Geometry: final body of the model. Coordinates: model frame, mm. A direction names the side the tool comes from. Give positions to 0.01 mm unless a question says otherwise; leave off trailing zeros. Order: outer loops, then holes, each group sorted by start corner. A loop starts at its lowest first (then second) coordinate and runs counter-clockwise, first axis right, second up. Notation, with made-up numbers: (37, -7) -> (46, -7) arc R24 ccw to (46, 18) -> close; hole circle Ø8 at (16, -38). An arc over 180 degrees is marked (long way). Write item = value, one per line.
```python
from build123d import *

# Parameters (mm, degrees)
SKETCH_1_W           = 174.15
SKETCH_1_H           = 108
EXTRUDE_1_DEPTH      = 63
CUT_EXTRUDE_2_DEPTH  = 174.15
CUT_EXTRUDE_3_REACH  = 122.279
SKETCH_6_W           = 2
SKETCH_6_H           = 108
SKETCH_7_W           = 96
SKETCH_7_H           = 50.25
CUT_EXTRUDE_5_DEPTH  = 168.15
SKETCH_8_W           = 87.5
SKETCH_8_H           = 4.75
CUT_EXTRUDE_6_DEPTH  = 168.15
SKETCH_10_W          = 168.15
SKETCH_10_H          = 87.5
CUT_EXTRUDE_8_DEPTH  = 59
SKETCH_12_W          = 168.15
SKETCH_12_H          = 96
EXTRUDE_2_DEPTH      = 2
SKETCH_15_W          = 25
SKETCH_15_H          = 70
SKETCH_15_W_2        = 55
SKETCH_15_H_2        = 20
SKETCH_15_W_3        = 44.398131355
SKETCH_15_H_3        = 87.5
CUT_EXTRUDE_9_DEPTH  = 2
SKETCH_16_W          = 25
SKETCH_16_H          = 96
SKETCH_16_W_2        = 32.283516817
CUT_EXTRUDE_10_DEPTH = 2
SKETCH_17_W          = 2
SKETCH_17_H          = 96
EXTRUDE_3_DEPTH      = 5
SKETCH_18_W          = 2
SKETCH_18_H          = 87.5
EXTRUDE_4_DEPTH      = 5
SKETCH_19_W          = 100
SKETCH_19_H          = 18
CUT_EXTRUDE_11_DEPTH = 6
CUT_EXTRUDE_12_REACH = 154.365
EXTRUDE_5_REACH      = 154.365
SKETCH_23_W          = 65.205598619
SKETCH_23_H          = 48.744694075
CUT_EXTRUDE_13_DEPTH = 2
CUT_EXTRUDE_START    = -63
CUT_EXTRUDE_14_DEPTH = 63
SKETCH_28_W          = 2
SKETCH_28_H          = 4.25
EXTRUDE_6_DEPTH      = 4.75
SKETCH_31_W          = 13
SKETCH_31_H          = 55
CUT_EXTRUDE_15_DEPTH = 10
SKETCH_34_W          = 103.070926165
SKETCH_34_H          = 3
CUT_EXTRUDE_16_DEPTH = 143.15
SKETCH_37_W          = 0.5
SKETCH_37_H          = 0.5
EXTRUDE_7_DEPTH      = 1
EXTRUDE_7_2_DEPTH    = 1
EXTRUDE_7_3_DEPTH    = 1
EXTRUDE_7_4_DEPTH    = 1
EXTRUDE_7_5_DEPTH    = 1
EXTRUDE_7_6_DEPTH    = 1
EXTRUDE_7_7_DEPTH    = 1
SKETCH_40_W          = 0.5
SKETCH_40_H          = 0.5
EXTRUDE_8_DEPTH      = 1
SKETCH_42_W          = 2.002594571
SKETCH_42_H          = 94
EXTRUDE_9_DEPTH      = 63


with BuildPart() as part:
    # Sketch 1 → Extrude 1 (new body)
    with BuildSketch(Plane(origin=(0, 0, 0), x_dir=(1, 0, 0), z_dir=(0, 1, 0))):
        Rectangle(SKETCH_1_W, SKETCH_1_H)
    extrude(amount=EXTRUDE_1_DEPTH)

    # Sketch 5 → Cut-Extrude 2 (cut)
    with BuildSketch(Plane.ZY.offset(87.075)):
        Polygon((-48, 0), (-47.75, 0), (-47.75, 2.75), (-45.75, 2.75), (-45.75, 4.75), (-52.25, 4.75), (-52.25, 2.75), (-50.25, 2.75), (-50.25, 0), (-50, 0), (-50, 3), (-52, 3), (-52, 4.5), (-46, 4.5), (-46, 3), (-48, 3), align=None)
        Polygon((-50, 0), (-48, 0), (-48, 3), (-46, 3), (-46, 4.5), (-52, 4.5), (-52, 3), (-50, 3), align=None)
        Polygon((50, 3), (50, 0), (50.25, 0), (50.25, 2.75), (52.25, 2.75), (52.25, 4.75), (45.75, 4.75), (45.75, 2.75), (47.75, 2.75), (47.75, 0), (48, 0), (48, 3), (46, 3), (46, 4.5), (52, 4.5), (52, 3), align=None)
        Polygon((48, 0), (50, 0), (50, 3), (52, 3), (52, 4.5), (46, 4.5), (46, 3), (48, 3), align=None)
    extrude(amount=-CUT_EXTRUDE_2_DEPTH, mode=Mode.SUBTRACT)

    # Cut-Extrude 3: up to this face of the body (flat: up to its plane)
    cut_extrude_3_end = Plane(part.part.faces().sort_by_distance((0, 4.75, 49))[0])
    # Sketch 6 → Cut-Extrude 3 (cut, up to the picked face)
    with BuildSketch(Plane.XZ, mode=Mode.PRIVATE) as cut_extrude_3_sk1:
        with Locations((-86.075, 0)):
            Rectangle(SKETCH_6_W, SKETCH_6_H)
    cut_extrude_3_tool1 = split(extrude(cut_extrude_3_sk1.sketch, amount=-CUT_EXTRUDE_3_REACH, mode=Mode.PRIVATE), bisect_by=cut_extrude_3_end, keep=Keep.BOTH, mode=Mode.PRIVATE)
    add(cut_extrude_3_tool1.solids().sort_by(Axis((-86.075, 0, 0), (0, 1, 0)))[0], mode=Mode.SUBTRACT)

    # Sketch 7 → Cut-Extrude 5 (cut)
    with BuildSketch(Plane(origin=(87.075, 0, 0), x_dir=(0, 0, -1), z_dir=(1, 0, 0))):
        with Locations((0, 31.875)):
            Rectangle(SKETCH_7_W, SKETCH_7_H)
    extrude(amount=-CUT_EXTRUDE_5_DEPTH, mode=Mode.SUBTRACT)

    # Sketch 8 → Cut-Extrude 6 (cut)
    with BuildSketch(Plane(origin=(87.075, 0, 0), x_dir=(0, 0, -1), z_dir=(1, 0, 0))):
        with Locations((0, 4.375)):
            Rectangle(SKETCH_8_W, SKETCH_8_H)
    extrude(amount=-CUT_EXTRUDE_6_DEPTH, mode=Mode.SUBTRACT)

    # Sketch 10 → Cut-Extrude 8 (cut)
    with BuildSketch(Plane(origin=(0, 2, 0), x_dir=(1, 0, 0), z_dir=(0, 1, 0))):
        with Locations((3, 0)):
            Rectangle(SKETCH_10_W, SKETCH_10_H)
    extrude(amount=CUT_EXTRUDE_8_DEPTH, mode=Mode.SUBTRACT)

    # Sketch 12 → Extrude 2 (add)
    with BuildSketch(Plane(origin=(0, 24, 0), x_dir=(-1, 0, 0), z_dir=(0, -1, 0))):
        with Locations((-3, 0)):
            Rectangle(SKETCH_12_W, SKETCH_12_H)
    extrude(amount=EXTRUDE_2_DEPTH)

    # Sketch 15 → Cut-Extrude 9 (cut)
    with BuildSketch(Plane(origin=(0, 2, 0), x_dir=(1, 0, 0), z_dir=(0, 1, 0))):
        with Locations((-68.575, 8.75)):
            Rectangle(SKETCH_15_W, SKETCH_15_H)
        with Locations((-9.233175572, -33.75)):
            Rectangle(SKETCH_15_W_2, SKETCH_15_H_2)
        with Locations((64.875934323, 0)):
            Rectangle(SKETCH_15_W_3, SKETCH_15_H_3)
    extrude(amount=-CUT_EXTRUDE_9_DEPTH, mode=Mode.SUBTRACT)

    # Sketch 16 → Cut-Extrude 10 (cut)
    with BuildSketch(Plane(origin=(0, 24, 0), x_dir=(1, 0, 0), z_dir=(0, 1, 0))):
        with Locations((-68.575, 0)):
            Rectangle(SKETCH_16_W, SKETCH_16_H)
        with Locations((70.933241592, 0)):
            Rectangle(SKETCH_16_W_2, SKETCH_16_H)
    extrude(amount=-CUT_EXTRUDE_10_DEPTH, mode=Mode.SUBTRACT)

    # Sketch 17 → Extrude 3 (add)
    with BuildSketch(Plane(origin=(0, 24, 0), x_dir=(1, 0, 0), z_dir=(0, 1, 0))):
        with Locations((-55.075, 0)):
            Rectangle(SKETCH_17_W, SKETCH_17_H)
    extrude(amount=EXTRUDE_3_DEPTH)

    # Sketch 18 → Extrude 4 (add)
    with BuildSketch(Plane(origin=(0, 2, 0), x_dir=(1, 0, 0), z_dir=(0, 1, 0))):
        with Locations((-55.075, 0)):
            Rectangle(SKETCH_18_W, SKETCH_18_H)
    extrude(amount=EXTRUDE_4_DEPTH)

    # Sketch 19 → Cut-Extrude 11 (cut)
    with BuildSketch(Plane(origin=(0, 0, 48), x_dir=(-1, 0, 0), z_dir=(0, 0, -1))):
        with Locations((4.075, 38)):
            Rectangle(SKETCH_19_W, SKETCH_19_H)
    extrude(amount=-CUT_EXTRUDE_11_DEPTH, mode=Mode.SUBTRACT)

    # Cut-Extrude 12: up to this face of the body (flat: up to its plane)
    cut_extrude_12_end = Plane(part.part.faces().sort_by_distance((0.074595533, 31.525240719, -54))[0])
    # Sketch 20 → Cut-Extrude 12 (cut, up to the picked face)
    with BuildSketch(Plane.XY.offset(54), mode=Mode.PRIVATE) as cut_extrude_12_sk1:
        Polygon((-87.075, 4.75), (-54.075, 63), (-87.075, 63), align=None)
    cut_extrude_12_tool1 = split(extrude(cut_extrude_12_sk1.sketch, amount=-CUT_EXTRUDE_12_REACH, mode=Mode.PRIVATE), bisect_by=cut_extrude_12_end, keep=Keep.BOTH, mode=Mode.PRIVATE)
    add(cut_extrude_12_tool1.solids().sort_by(Axis((-76.075, 43.583333, 54), (0, 0, -1)))[0], mode=Mode.SUBTRACT)

    # Extrude 5: up to this face of the body (flat: up to its plane)
    extrude_5_end = Plane(part.part.faces().sort_by_distance((7.392919772, 30.366402897, -54))[0])
    # Sketch 21 → Extrude 5 (add, up to the picked face)
    with BuildSketch(Plane.XY.offset(54), mode=Mode.PRIVATE) as extrude_5_sk1:
        Polygon((-87.075, 4.75), (-84.776349095, 4.75), (-51.776349095, 63), (-54.075, 63), align=None)
    extrude_5_tool1 = split(extrude(extrude_5_sk1.sketch, amount=-EXTRUDE_5_REACH, mode=Mode.PRIVATE), bisect_by=extrude_5_end, keep=Keep.BOTH, mode=Mode.PRIVATE)
    add(extrude_5_tool1.solids().sort_by(Axis((-69.425675, 33.875, 54), (0, 0, -1)))[0])

    # Sketch 23 → Cut-Extrude 13 (cut)
    with BuildSketch(Plane(origin=(0, 63, 0), x_dir=(1, 0, 0), z_dir=(0, 1, 0))):
        with Locations((-5.140341164, 12.481591832)):
            Rectangle(SKETCH_23_W, SKETCH_23_H)
    extrude(amount=-CUT_EXTRUDE_13_DEPTH, mode=Mode.SUBTRACT)

    # Sketch 26 → Cut-Extrude 14 (cut)
    with BuildSketch(Plane(origin=(0, 63, 0), x_dir=(1, 0, 0), z_dir=(0, 1, 0)).offset(CUT_EXTRUDE_START)):
        Polygon((82.075, 52), (85.075, 52), (85.075, 48), (87.075, 48), (87.075, -48), (85.075, -48), (85.075, -52), (82.075, -52), align=None)
    extrude(amount=CUT_EXTRUDE_14_DEPTH, mode=Mode.SUBTRACT)

    # Sketch 28 → Extrude 6 (add)
    with BuildSketch(Plane.XZ.offset(-4.75)):
        with Locations((86.075, 50.125)):
            Rectangle(SKETCH_28_W, SKETCH_28_H)
        with Locations((86.075, -50.125)):
            Rectangle(SKETCH_28_W, SKETCH_28_H)
    extrude(amount=EXTRUDE_6_DEPTH)

    # Sketch 31 → Cut-Extrude 15 (cut)
    with BuildSketch(Plane(origin=(0, 63, 0), x_dir=(1, 0, 0), z_dir=(0, 1, 0))):
        with Locations((75.575, 0)):
            Rectangle(SKETCH_31_W, SKETCH_31_H)
    extrude(amount=-CUT_EXTRUDE_15_DEPTH, mode=Mode.SUBTRACT)

    # Sketch 34 → Cut-Extrude 16 (cut)
    with BuildSketch(Plane(origin=(87.075, 0, 0), x_dir=(0, 0, -1), z_dir=(1, 0, 0))):
        with Locations((-0.464536917, 23.5)):
            Rectangle(SKETCH_34_W, SKETCH_34_H)
    extrude(amount=-CUT_EXTRUDE_16_DEPTH, mode=Mode.SUBTRACT)

    # Sketch 40 → Extrude 8 (add)
    with BuildSketch(Plane.XY.offset(-48)):
        with Locations((86.075, 61.396326998)):
            Rectangle(SKETCH_40_W, SKETCH_40_H)
        with Locations((86.075, 51.396326998)):
            Rectangle(SKETCH_40_W, SKETCH_40_H)
        with Locations((86.075, 41.396326998)):
            Rectangle(SKETCH_40_W, SKETCH_40_H)
        with Locations((86.075, 31.396326998)):
            Rectangle(SKETCH_40_W, SKETCH_40_H)
        with Locations((86.075, 21.396326998)):
            Rectangle(SKETCH_40_W, SKETCH_40_H)
        with Locations((86.075, 11.396326998)):
            Rectangle(SKETCH_40_W, SKETCH_40_H)
        with Locations((86.075, 1.396326998)):
            Rectangle(SKETCH_40_W, SKETCH_40_H)
    extrude(amount=EXTRUDE_8_DEPTH)



with BuildPart() as body_2:
    # Sketch 37 → Extrude 7 (new body)
    with BuildSketch(Plane(origin=(0, 0, 48), x_dir=(-1, 0, 0), z_dir=(0, 0, -1))):
        with Locations((-86.075, 51.75934634)):
            Rectangle(SKETCH_37_W, SKETCH_37_H)
    extrude(amount=EXTRUDE_7_DEPTH)


with BuildPart() as body_3:
    # Sketch 37 → Extrude 7 2 (new body)
    with BuildSketch(Plane(origin=(0, 0, 48), x_dir=(-1, 0, 0), z_dir=(0, 0, -1))):
        with Locations((-86.075, 61.75934634)):
            Rectangle(SKETCH_37_W, SKETCH_37_H)
    extrude(amount=EXTRUDE_7_2_DEPTH)


with BuildPart() as body_4:
    # Sketch 37 → Extrude 7 3 (new body)
    with BuildSketch(Plane(origin=(0, 0, 48), x_dir=(-1, 0, 0), z_dir=(0, 0, -1))):
        with Locations((-86.075, 41.75934634)):
            Rectangle(SKETCH_37_W, SKETCH_37_H)
    extrude(amount=EXTRUDE_7_3_DEPTH)


with BuildPart() as body_5:
    # Sketch 37 → Extrude 7 4 (new body)
    with BuildSketch(Plane(origin=(0, 0, 48), x_dir=(-1, 0, 0), z_dir=(0, 0, -1))):
        with Locations((-86.075, 31.75934634)):
            Rectangle(SKETCH_37_W, SKETCH_37_H)
    extrude(amount=EXTRUDE_7_4_DEPTH)


with BuildPart() as body_6:
    # Sketch 37 → Extrude 7 5 (new body)
    with BuildSketch(Plane(origin=(0, 0, 48), x_dir=(-1, 0, 0), z_dir=(0, 0, -1))):
        with Locations((-86.075, 21.75934634)):
            Rectangle(SKETCH_37_W, SKETCH_37_H)
    extrude(amount=EXTRUDE_7_5_DEPTH)


with BuildPart() as body_7:
    # Sketch 37 → Extrude 7 6 (new body)
    with BuildSketch(Plane(origin=(0, 0, 48), x_dir=(-1, 0, 0), z_dir=(0, 0, -1))):
        with Locations((-86.075, 11.75934634)):
            Rectangle(SKETCH_37_W, SKETCH_37_H)
    extrude(amount=EXTRUDE_7_6_DEPTH)


with BuildPart() as body_8:
    # Sketch 37 → Extrude 7 7 (new body)
    with BuildSketch(Plane(origin=(0, 0, 48), x_dir=(-1, 0, 0), z_dir=(0, 0, -1))):
        with Locations((-86.075, 1.75934634)):
            Rectangle(SKETCH_37_W, SKETCH_37_H)
    extrude(amount=EXTRUDE_7_7_DEPTH)


with BuildPart() as part_1:
    add(part.part)

    add(body_2.part)  # Extrude 9 merges body 2

    add(body_3.part)  # Extrude 9 merges body 3

    add(body_4.part)  # Extrude 9 merges body 4

    add(body_5.part)  # Extrude 9 merges body 5

    add(body_6.part)  # Extrude 9 merges body 6

    add(body_7.part)  # Extrude 9 merges body 7

    add(body_8.part)  # Extrude 9 merges body 8
    # Sketch 42 → Extrude 9 (add)
    with BuildSketch(Plane(origin=(0, 63, 0), x_dir=(1, 0, 0), z_dir=(0, 1, 0))):
        with Locations((86.076297286, 0)):
            Rectangle(SKETCH_42_W, SKETCH_42_H)
    extrude(amount=-EXTRUDE_9_DEPTH)


solid = part_1.part
```
1) First-contact query: P1, Ø0.6, axis at x = 86, z = 47.5, coming from the -Y side; P2, Ø5, axis at x = -74, z = 34.5, coming from the +Y side; P3, Ø0.6, axis at x = 86, z = -47.5, coming from the +Y side; P4, Ø1.3, axis at x = -10.5, z = -45, coming from the -Y side. Flat tips, straight axial feed; report the tip coordinate or a pass-through.
Check sheet entries:
P1 = 1.51
P2 = 32.24
P3 = 61.65
P4 = 0
2) Section query B-B (z = 17.5). Output: boundary loops of the cut face in (x, y) (3 decimals).
Check sheet entries:
outline = (-87.075, 4.75) -> (-85.075, 4.75) -> (-85.075, 0) -> (-81.075, 0) -> (-81.075, 11.283) -> (-52.909, 61) -> (69.075, 61) -> (69.075, 63) -> (-54.075, 63) -> close; (-56.075, 0) -> (42.677, 0) -> (42.677, 2) -> (-54.075, 2) -> (-54.075, 7) -> (-56.075, 7) -> close; (-56.075, 25) -> (-54.075, 25) -> (-54.075, 29) -> (-56.075, 29) -> close; (85.075, 0) -> (87.078, 0) -> (87.078, 63) -> (85.075, 63) -> close
3) Line query: line 1 (Y direction, x = 10, z = 12); line 2 (Z direction, x = 33, y = 49); line 3 (X direction, y = 6, z = -5.5) (3 decimals). Output: solid intervals per line, ascending. Write a range as from..to.
Check sheet entries:
line_1 = 0..2, 61..63
line_2 = -54..-48, 48..54
line_3 = -86.367..-81.075, -56.075..-54.075, 85.075..87.078
4) Section query C-C (x = -18.5). Count the separate pieces of the cut face and the enclosed holes in it, plus the area to 3 significant figures.
Check sheet entries:
separate_pieces = 3
enclosed_holes = 0
area = 908 mm²
5) Reachability of faces 1 (the face through (-69, 4, 43.75)), 2 (the face through (-54.075, 38, 51)), 3 (the face through (-68, 3, -43.75)), 4 (the face through (82.075, 48, 49)) from +Z, -Z, +X, -X, +Y, -Y: full face, straight path, thin tool, end or side. Return the list, or none.
Check sheet entries:
face_1 = none
face_2 = +Z
face_3 = -Y
face_4 = +Y, -Y
6) Section query D-D (y = 35.5). Output: boundary loops of the cut face in (x, z) (3 decimals), plus the area to 3 significant figures.
Check sheet entries:
outline = (-69.654, -54) -> (87.075, -54) -> (87.075, -48) -> (85.075, -48) -> (85.075, -52) -> (82.075, -52) -> (82.075, -48) -> (-67.356, -48) -> (-67.356, 48) -> (-54.075, 48) -> (-54.075, 54) -> (-69.654, 54) -> close; (45.925, 48) -> (82.075, 48) -> (82.075, 52) -> (85.075, 52) -> (85.075, 48) -> (87.075, 48) -> (87.075, 54) -> (45.925, 54) -> close; (85.075, -47) -> (87.078, -47) -> (87.078, 47) -> (85.075, 47) -> close
area = 1,670 mm²
7) Section query A-A (z = -34). Output: boundary loops of the cut face in (x, y) (3 decimals), plus the area to 3 significant figures.
Check sheet entries:
outline = (-87.075, 4.75) -> (-85.075, 4.75) -> (-85.075, 0) -> (-81.075, 0) -> (-81.075, 11.283) -> (-52.909, 61) -> (-37.743, 61) -> (-37.743, 63) -> (-54.075, 63) -> close; (-56.075, 0) -> (42.677, 0) -> (42.677, 2) -> (-54.075, 2) -> (-54.075, 7) -> (-56.075, 7) -> close; (-56.075, 25) -> (-54.075, 25) -> (-54.075, 29) -> (-56.075, 29) -> close; (27.462, 61) -> (82.075, 61) -> (82.075, 63) -> (27.462, 63) -> close; (85.075, 0) -> (87.078, 0) -> (87.078, 63) -> (85.075, 63) -> close
area = 645 mm²
8) Mould query, pull axis X, two halves, no side actions, for faces 5 (the face through (14, 22, 50)), 6 (the face through (-85.075, 2, -1)), 7 (the face through (-56.075, 27, 1)). Classes: +X half, -X half, draft (parallel to the pull), parting line (faces both ways), or undercut.
Check sheet entries:
face_5 = draft
face_6 = -X half
face_7 = undercut
